Read the model definition and answer for the solid it produces. Units are mm, in the model's axes. Give positions to 0.01 mm unless a question says otherwise; leave off trailing zeros. Order: outer loops, then holes, each group sorted by start corner. A loop starts at its lowest first (then second) coordinate and runs counter-clockwise, first axis right, second up. Notation, with made-up numbers: (44, -1) - (50, -1) arc R21 cw to (50, 29) - close; hole circle Ø11 at (78.5, -23). An arc over 180 degrees is marked (long way). Return JSON: item names as keys, results as strings.
```python
from build123d import *

# Parameters (mm, degrees)
SKETCH1_W           = 250
SKETCH1_H           = 250
BOSS_EXTRUDE1_DEPTH = 2
SKETCH2_R           = 10.5
CUT_EXTRUDE1_DEPTH  = 177.788008643


with BuildPart() as part:
    # Sketch1 → Boss-Extrude1 (new body)
    with BuildSketch(Plane(origin=(0, 0, 0), x_dir=(1, 0, 0), z_dir=(0, 1, 0))):
        Rectangle(SKETCH1_W, SKETCH1_H)
    extrude(amount=BOSS_EXTRUDE1_DEPTH)

    # Sketch2 → Cut-Extrude1 (cut, through all)
    with BuildSketch(Plane(origin=(0, 2, 0), x_dir=(1, 0, 0), z_dir=(0, 1, 0))):
        with Locations(Location((-100, 100, 0), (0, 0, 270))):
            Circle(SKETCH2_R)
        with Locations(Location((-50, 100, 0), (0, 0, 270))):
            Circle(SKETCH2_R)
        with Locations(Location((0, 100, 0), (0, 0, 270))):
            Circle(SKETCH2_R)
        with Locations(Location((50, 100, 0), (0, 0, 270))):
            Circle(SKETCH2_R)
        with Locations(Location((100, 100, 0), (0, 0, 270))):
            Circle(SKETCH2_R)
        with Locations(Location((-50, 50, 0), (0, 0, 270))):
            Circle(SKETCH2_R)
        with Locations(Location((0, 50, 0), (0, 0, 270))):
            Circle(SKETCH2_R)
        with Locations(Location((50, 50, 0), (0, 0, 270))):
            Circle(SKETCH2_R)
        with Locations(Location((100, 50, 0), (0, 0, 270))):
            Circle(SKETCH2_R)
        with Locations(Location((-50, 0, 0), (0, 0, 270))):
            Circle(SKETCH2_R)
        with Locations(Location((0, 0, 0), (0, 0, 270))):
            Circle(SKETCH2_R)
        with Locations(Location((50, 0, 0), (0, 0, 270))):
            Circle(SKETCH2_R)
        with Locations(Location((100, 0, 0), (0, 0, 270))):
            Circle(SKETCH2_R)
        with Locations(Location((-50, -50, 0), (0, 0, 270))):
            Circle(SKETCH2_R)
        with Locations(Location((0, -50, 0), (0, 0, 270))):
            Circle(SKETCH2_R)
        with Locations(Location((50, -50, 0), (0, 0, 270))):
            Circle(SKETCH2_R)
        with Locations(Location((100, -50, 0), (0, 0, 270))):
            Circle(SKETCH2_R)
        with Locations(Location((-50, -100, 0), (0, 0, 270))):
            Circle(SKETCH2_R)
        with Locations(Location((0, -100, 0), (0, 0, 270))):
            Circle(SKETCH2_R)
        with Locations(Location((50, -100, 0), (0, 0, 270))):
            Circle(SKETCH2_R)
        with Locations(Location((100, -100, 0), (0, 0, 270))):
            Circle(SKETCH2_R)
        with Locations(Location((-100, 50, 0), (0, 0, 270))):
            Circle(SKETCH2_R)
        with Locations(Location((-100, 0, 0), (0, 0, 270))):
            Circle(SKETCH2_R)
        with Locations(Location((-100, -50, 0), (0, 0, 270))):
            Circle(SKETCH2_R)
        with Locations(Location((-100, -100, 0), (0, 0, 270))):
            Circle(SKETCH2_R)
    extrude(amount=-CUT_EXTRUDE1_DEPTH, mode=Mode.SUBTRACT)


solid = part.part
```
Q1. A cutting plane is placed at B-B (y = 0.8). Give the number of separate pieces and of enclosed holes in the cut face, and give its area (3 significant figures).
Values:
{"separate pieces": "1", "enclosed holes": "25", "area": "53,800 mm²"}
Q2. A cutting plane is placed at A-A (z = -50). Write down the section's boundary in (x, y).
Values:
{"outline": "(-125, 0) - (-110.5, 0) - (-110.5, 2) - (-125, 2) - close; (-89.5, 0) - (-60.5, 0) - (-60.5, 2) - (-89.5, 2) - close; (-39.5, 0) - (-10.5, 0) - (-10.5, 2) - (-39.5, 2) - close; (10.5, 0) - (39.5, 0) - (39.5, 2) - (10.5, 2) - close; (60.5, 0) - (89.5, 0) - (89.5, 2) - (60.5, 2) - close; (110.5, 0) - (125, 0) - (125, 2) - (110.5, 2) - close"}
Q3. Given pin 1 (17 mm diameter, centred on x = 50, z = -50, fed in from +Y); pin 2 (3 mm diameter, centred on x = 21, z = 48.5, fed in from -Y), each flat-ended and moving along its own axis, determine where each tip first touches the part or whether it passes through.
Values:
{"pin 1": "passes through", "pin 2": "stops at y = 0"}
Q4. Consider L1, parallel to X at y = 1, z = 100; L2, parallel to X at y = 0.5, z = -54; L3, parallel to Z at x = -51.5, y = 1.9. Determine where each line is inside the solid, lowest interval first.
Values:
{"L1": "x = -125 to -110.5, -89.5 to -60.5, -39.5 to -10.5, 10.5 to 39.5, 60.5 to 89.5, 110.5 to 125", "L2": "x = -125 to -109.71, -90.29 to -59.71, -40.29 to -9.71, 9.71 to 40.29, 59.71 to 90.29, 109.71 to 125", "L3": "z = -125 to -110.39, -89.61 to -60.39, -39.61 to -10.39, 10.39 to 39.61, 60.39 to 89.61, 110.39 to 125"}
Q5. Determine the mould class of faces 1 (the cylindrical face through (-92.904, 1.014, -57.739)), 2 (the flat face through (-30, 2, -2)) for opening direction X: released by +X, released by -X, zero draft, split by the parting line, or undercut.
Values:
{"face 1": "undercut", "face 2": "zero draft"}
Q6. A cutting plane is placed at C-C (x = 0). Write down the section's boundary in (y, z).
Values:
{"outline": "(0, -125) - (2, -125) - (2, -110.5) - (0, -110.5) - close; (0, -89.5) - (2, -89.5) - (2, -60.5) - (0, -60.5) - close; (0, -39.5) - (2, -39.5) - (2, -10.5) - (0, -10.5) - close; (0, 10.5) - (2, 10.5) - (2, 39.5) - (0, 39.5) - close; (0, 60.5) - (2, 60.5) - (2, 89.5) - (0, 89.5) - close; (0, 110.5) - (2, 110.5) - (2, 125) - (0, 125) - close"}
